The listing builds one solid part. Answer for the finished solid, in the listing's coordinates (mm). A direction names the side the tool comes from. Give positions to 0.01 mm unless a question says otherwise; leave off trailing zeros. Loops run counter-clockwise (first coordinate to the right, second up) from the corner with the lowest first, then second, coordinate; pieces in that order, holes last. Notation, with made-up numbers: (-29, 44) - (-7, 44) arc R26 cw to (-7, 63) - close; hole circle Ø11 at (8, 46.25). An arc over 180 degrees is marked (long way). Answer as CSV lines item,"result". Start each with the question number.
1) Find the intervals of material crossed by line 1 along Y through (x, z) = (-0.5, 31.5) (1 decimal); line 2 along Y through (x, z) = (0, 17) (3 decimals); line 3 along Z through (x, y) = (-7, 7.5) (3 decimals), in increasing order.
2) For a pull along Z with two mould halves and no side action, classify faces 4 (the face through (9.67, 5.48, 4.7)), 5 (the face through (0, 12, 44.45)), 6 (the face through (0, 11.112, 33)), 7 (the face through (0, 10, 39.688)) as pulls with the +Z half, pulls with the -Z half, needs draft (parallel to the pull), parting line crosses it, or undercut.
3) A cutting plane is placed at D-D (y = -7.5). Determine the outline of the cut face in (x, z) (3 decimals), and give its area (3 significant figures).
4) For faces 1 (the face through (0, 14, 26.988)), 2 (the face through (6.35, 12, 38)), 3 (the face through (4, 9, 9.525)), determine the directions among +Z, -Z, +X, -X, +Y, -Y from which every point of the face is accessible in a straight line to the end or side of a thin tool.
5) Flat-ended cylindrical pins translate along their axes: pin 1 (5 mm diameter, centred on x = -7, z = 41.5, fed in from -Y) (3 decimals); pin 2 (2.5 mm diameter, centred on y = 12, z = 35, fed in from -X); pin 3 (7 mm diameter, centred on y = 12, z = 39.5, fed in from +X); pin 4 (6 mm diameter, centred on x = -5.5, z = -2.5, fed in from -Y). Find the tip coordinate at first contact, or state that the pin passes through.
```python
from build123d import *

# Parameters (mm, degrees)
BOSS_EXTRUDE1_DEPTH      = 9.525
SKETCH2_R                = 5.1054
BOSS_EXTRUDE2_DEPTH      = 9.525
BOSS_EXTRUDE2_TAPER      = 3.5
SKETCH3_R                = 9.525
BOSS_EXTRUDE3_DEPTH      = 38.1
BOSS_EXTRUDE5_DEPTH      = 6.35
BOSS_EXTRUDE5_DEPTH_BACK = 9.525
SKETCH5_W                = 12.7
SKETCH5_H                = 4.7625
SKETCH6_W                = 12.7
SKETCH6_H                = 4.7625
BOSS_EXTRUDE6_DEPTH      = 12.7


with BuildPart() as part:
    # Sketch1 → Boss-Extrude1 (new body)
    with BuildSketch(Plane.XY):
        Polygon((6.415804866, 11.1125), (-6.415804866, 11.1125), (-12.831609733, 0), (-6.415804866, -11.1125), (6.415804866, -11.1125), (12.831609733, 0), align=None)
    extrude(amount=BOSS_EXTRUDE1_DEPTH)

    # Sketch2 → Boss-Extrude2 (add)
    with BuildSketch(Plane(origin=(0, 0, 0), x_dir=(-1, 0, 0), z_dir=(0, 0, -1))):
        Circle(SKETCH2_R)
    extrude(amount=BOSS_EXTRUDE2_DEPTH, taper=BOSS_EXTRUDE2_TAPER)

    # Sketch3 → Boss-Extrude3 (add)
    with BuildSketch(Plane.XY.offset(9.525)):
        with Locations(Location((0, 0, 0), (0, 0, 180))):
            Circle(SKETCH3_R)
    extrude(amount=BOSS_EXTRUDE3_DEPTH)

    # Sketch5 → Boss-Extrude5 (add, two sides: drawn at the far end of the back side and taken through both)
    with BuildSketch(Plane(origin=(0, 9.525, 0), x_dir=(1, 0, 0), z_dir=(0, 1, 0)).offset(-BOSS_EXTRUDE5_DEPTH_BACK)):
        with Locations((0, -42.06875)):
            Rectangle(SKETCH5_W, SKETCH5_H)
    extrude(amount=BOSS_EXTRUDE5_DEPTH + BOSS_EXTRUDE5_DEPTH_BACK)

    # Sketch6 → Boss-Extrude6 (add)
    with BuildSketch(Plane(origin=(0, 0, 39.6875), x_dir=(-1, 0, 0), z_dir=(0, 0, -1))):
        with Locations((0, 13.49375)):
            Rectangle(SKETCH6_W, SKETCH6_H)
    extrude(amount=BOSS_EXTRUDE6_DEPTH)


solid = part.part
```
Ans:
1,line 1,"-9.5 to 9.5, 11.1 to 15.9"
1,line 2,"-9.525 to 9.525"
1,line 3,"0 to 9.525"
2,face 4,"needs draft"
2,face 5,"pulls with the +Z half"
2,face 6,"undercut"
2,face 7,"undercut"
3,outline,"(-8.501, 0) - (8.501, 0) - (8.501, 9.525) - (5.872, 9.525) - (5.872, 47.625) - (-5.872, 47.625) - (-5.872, 9.525) - (-8.501, 9.525) - close"
3,area,"609 mm2"
4,face 1,"-Z, +X, -X, +Y"
4,face 2,"+Z, +X, +Y"
4,face 3,"none"
5,pin 1,"y = -8.395"
5,pin 2,"x = -6.35"
5,pin 3,"x = 6.35"
5,pin 4,"y = -11.11"
